from build123d import *

# Parameters (mm, degrees)
BOSS_EXTRUDE1_DEPTH = 0.1
BOSS_EXTRUDE2_DEPTH = 10


with BuildPart() as part:
    # Sketch1 → Boss-Extrude1 (new body)
    with BuildSketch(Plane.XY):
        with BuildLine():
            Line((-1544.649956659, 573.44143308), (-1542.397344254, 523.492201481))
            Line((-1542.397344254, 523.492201481), (-1721.722963635, 515.404967666))
            Line((-1721.722963635, 515.404967666), (-1723.97557604, 565.354199265))
            Line((-1723.97557604, 565.354199265), (-1743.607960183, 593.830470178))
            add(Edge.make_bspline(
                [(-1743.607960183, 593.830470178), (-1719.507904213, 610.537812828), (-1709.389541143, 613.399774739), (-1646.280289738, 619.241808081), (-1585.716648888, 600.423930323), (-1544.649956659, 573.44143308)],
                knots=[0, 0, 0, 0, 0.320554642, 0.420554642, 1, 1, 1, 1], degree=3))
        make_face()
    extrude(amount=BOSS_EXTRUDE1_DEPTH)

    # Sketch2 → Boss-Extrude2 (add)
    with BuildSketch(Plane.XY.offset(0.1)):
        with BuildLine():
            Line((-1544.677412579, 573.399645851), (-1544.732324417, 573.316071394))
            add(Edge.make_bspline(
                [(-1544.732324417, 573.316071394), (-1546.951948835, 574.774455463), (-1551.43127801, 577.613556033), (-1560.629429442, 583.045346231), (-1572.470935952, 589.326889692), (-1587.069867375, 596.019330748), (-1606.812651261, 603.755089396), (-1626.620904389, 609.625271881), (-1645.785452529, 613.461587482), (-1659.664022733, 615.275078476), (-1672.855430865, 616.000525973), (-1683.17584634, 615.607177853), (-1690.719151522, 614.940047919), (-1697.619410573, 614.184343593), (-1704.94143994, 613.175751133), (-1711.537062872, 611.520585877), (-1716.950731756, 609.496349748), (-1721.226339774, 607.54713974), (-1725.861820037, 605.087085053), (-1730.144377714, 602.544994912), (-1733.894814235, 600.175895508), (-1736.886084267, 598.222624564), (-1739.548362017, 596.435520579), (-1741.775682708, 594.914415574), (-1742.945821332, 594.106977842), (-1743.522500251, 593.707195687)],
                knots=[0, 0, 0, 0, 0.03125, 0.0625, 0.125, 0.1875, 0.25, 0.375, 0.4375, 0.5, 0.5625, 0.625, 0.65625, 0.6875, 0.75, 0.8125, 0.84375, 0.875, 0.90625, 0.9375, 0.953125, 0.96875, 0.984375, 0.9921875, 1, 1, 1, 1], degree=3))
            Line((-1743.522500251, 593.707195687), (-1743.579473539, 593.789378681))
            add(Edge.make_bspline(
                [(-1544.677412579, 573.399645851), (-1580.106306882, 596.677879158), (-1623.417276611, 611.817205851), (-1664.055554326, 615.615316249), (-1668.458587485, 615.853546332), (-1674.850456886, 615.924640206), (-1676.947072346, 615.898899542), (-1681.053950245, 615.760083504), (-1685.070934683, 615.538033819), (-1688.841535286, 615.206941309), (-1692.455660822, 614.85004283), (-1694.182553399, 614.660043123), (-1699.092177305, 614.084892783), (-1702.026740338, 613.678931579), (-1710.391454065, 612.076086015), (-1715.382812403, 610.494610736), (-1727.278520434, 604.6086441), (-1734.182625539, 600.30373531), (-1743.579473539, 593.789378681)],
                knots=[0, 0, 0, 0, 0.5, 0.5, 0.5625, 0.5625, 0.59375, 0.59375, 0.625, 0.65625, 0.65625, 0.6875, 0.6875, 0.75, 0.75, 0.875, 0.875, 1, 1, 1, 1], degree=3))
        make_face()
    extrude(amount=BOSS_EXTRUDE2_DEPTH)


solid = part.part
CAD build for the part. Positions are in the model's coordinates, mm. Give positions to 0.01 mm unless a question says otherwise; leave off trailing zeros. Write each loop counter-clockwise with the first axis right and the second up, starting at its lowest first coordinate (ties: lowest second). Pieces come first, ordered by that corner, then holes. Notation, with made-up numbers: (-18.75, -3) - (23.25, -3) arc R25 cw to (23.25, 25) - close; hole circle Ø11 at (32, 11). An arc over 180 degrees is marked (long way). Put each result on its own line as item: value.
(1) Saw through at A-A (y = 546). List the corners of the cut face in (x, z), then the cut area to 3 significant figures.
Working result:
outline: (-1723.1, 0) - (-1543.41, 0) - (-1543.41, 0.1) - (-1723.1, 0.1) - close
area: 18.0 mm^2
(2) Wall check: L1, parallel to X at y = 597.5, z = 5.75; L2, parallel to X at y = 598, z = 5; L3, parallel to X at y = 583.5, z = 1.75. Give the ranges that are in metal, low to high.
Working result:
L1: -1738.14 to -1737.96, -1591.02 to -1590.76
L2: -1737.39 to -1737.21, -1592.26 to -1591.99
L3: -1561.65 to -1561.44
(3) Drop flat-ended pins along their axis: pin 1 Ø2 at (y, z) = (590.5, 9) entering from +X; pin 2 Ø1 at (x, z) = (-1571, 2.5) entering from -Y; pin 3 Ø1 at (x, y) = (-1657, 575) entering from +Z. Give the stop position or say it passes through.
Working result:
pin 1: x = -1572.95
pin 2: y = 588.17
pin 3: z = 0.1
